Read the model definition and answer for the solid it produces. Units are mm, in the model's axes. Face numbers are marked on the shaded views. A direction names the side the tool comes from. Give positions to 0.01 mm unless a question says otherwise; leave off trailing zeros. Order: outer loops, then holes, each group sorted by start corner. A loop starts at its lowest first (then second) coordinate and runs counter-clockwise, first axis right, second up. Notation, with made-up numbers: (-36, -13.75) - (-24, -13.75) arc R28 cw to (-24, 24.25) - close; hole circle Ø8 at (62.25, 36.5). An arc over 180 degrees is marked (long way). Return JSON: item names as keys, results as strings.
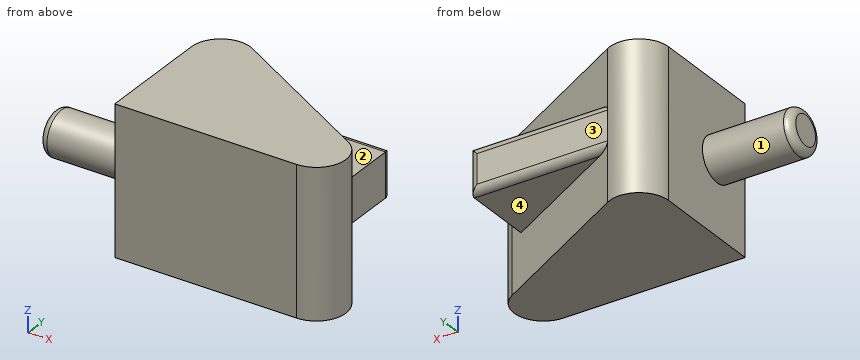
```python
from build123d import *

# Parameters (mm, degrees)
BOSS_EXTRUDE1_DEPTH = 5
SKETCH2_W           = 6.952682296
SKETCH2_H           = 2.551538718
SKETCH2_R           = 0.75
CUT_EXTRUDE1_DEPTH  = 3
SKETCH3_W           = 4.68163698
SKETCH3_H           = 1.5
BOSS_EXTRUDE2_DEPTH = 4.757403
FILLET1_R           = 0.25
FILLET2_R           = 0.25


with BuildPart() as part:
    # Sketch1 → Boss-Extrude1 (new body)
    with BuildSketch(Plane.XY):
        with BuildLine():
            Line((0, 2.17), (-3, 2.17))
            Line((-3, 2.17), (-3, 0.67))
            Line((-3, 0.67), (0, 0.67))
            Line((0, 0.67), (0, 0))
            Line((0, 0), (6.168897591, 0))
            ThreePointArc((6.168897591, 0), (7.13669318, 0.748262641), (6.656158202, 1.873256604))
            Line((6.656158202, 1.873256604), (1.487260611, 4.757403357))
            ThreePointArc((1.487260611, 4.757403357), (0.49367037, 4.74648677), (0, 3.884146753))
            Line((0, 3.884146753), (0, 2.17))
        make_face()
    extrude(amount=BOSS_EXTRUDE1_DEPTH)

    # Sketch2 → Cut-Extrude1 (cut)
    with BuildSketch(Plane.ZY.offset(3)):
        with Locations((2.401285903, 1.467822219)):
            Rectangle(SKETCH2_W, SKETCH2_H)
        with Locations((2.5, 1.42)):
            Circle(SKETCH2_R, mode=Mode.SUBTRACT)
    extrude(amount=-CUT_EXTRUDE1_DEPTH, mode=Mode.SUBTRACT)

    # Sketch3 → Boss-Extrude2 (add)
    with BuildSketch(Plane.XZ):
        with Locations((3.828079101, 2.5)):
            Rectangle(SKETCH3_W, SKETCH3_H)
    extrude(amount=-BOSS_EXTRUDE2_DEPTH)

    # Fillet1
    fillet1_edges = [part.edges().sort_by_distance(p)[0] for p in [
        (-3, 1.42, 1.75),
    ]]
    fillet(fillet1_edges, radius=FILLET1_R)

    # Fillet2
    fillet2_edges = [part.edges().sort_by_distance(p)[0] for p in [
        (3.828079101, 4.757403, 1.75),
        (3.828079101, 4.757403, 3.25),
        (6.168897591, 4.757403, 2.5),
    ]]
    fillet(fillet2_edges, radius=FILLET2_R)


solid = part.part
```
Q1. A cutting plane is placed at A-A (z = 1.3). Write down the section's boundary in (x, y).
Values:
{"outline": "(0, 0) - (6.17, 0) arc R1 ccw to (6.66, 1.87) - (1.49, 4.76) arc R1 ccw to (0, 3.88) - close"}
Q2. A cutting plane is placed at D-D (z = 2.5). Write down the section's boundary in (x, y).
Values:
{"outline": "(-3, 0.92) arc R0.25 ccw to (-2.75, 0.67) - (0, 0.67) - (0, 0) - (6.17, 0) arc R1 ccw to (6.66, 1.87) - (6.17, 2.15) - (6.17, 4.51) arc R0.25 ccw to (5.92, 4.76) - (1.49, 4.76) arc R1 ccw to (0, 3.88) - (0, 2.17) - (-2.75, 2.17) arc R0.25 ccw to (-3, 1.92) - close"}
Q3. Consider L1, parallel to Y at x = 4.5, z = 2.35; L2, parallel to X at y = 2.25, z = 1.9; L3, parallel to X at y = 2, z = 3.75. Determine where each line is inside the solid, lowest interval first.
Values:
{"L1": "y = 0 to 4.76", "L2": "x = 0 to 6.17", "L3": "x = 0 to 6.43"}
Q4. A cutting plane is placed at C-C (y = 1.42). Write down the section's boundary in (x, z).
Values:
{"outline": "(-3, 2) arc R0.25 ccw to (-2.75, 1.75) - (0, 1.75) - (0, 0) - (7.08, 0) - (7.08, 5) - (0, 5) - (0, 3.25) - (-2.75, 3.25) arc R0.25 ccw to (-3, 3) - close"}
Q5. A cutting plane is placed at B-B (x = 3.75). Write down the section's boundary in (y, z), and give its area (3 significant figures).
Values:
{"outline": "(0, 0) - (3.49, 0) - (3.49, 1.75) - (4.51, 1.75) arc R0.25 ccw to (4.76, 2) - (4.76, 3) arc R0.25 ccw to (4.51, 3.25) - (3.49, 3.25) - (3.49, 5) - (0, 5) - close", "area": "19.3 mm²"}
Q6. Given pin 1 (2 mm diameter, centred on x = 5, z = 2.5, fed in from +Y); pin 2 (1.2 mm diameter, centred on y = 4, z = 2.5, fed in from +X); pin 3 (1.2 mm diameter, centred on y = 2, z = 2, fed in from -X), each flat-ended and moving along its own axis, determine where each tip first touches the part or whether it passes through.
Values:
{"pin 1": "stops at y = 4.76", "pin 2": "stops at x = 6.17", "pin 3": "stops at x = -3"}
Q7. For the marked faces 1, 2, 3 and 4, determine the directions among +Z, -Z, +X, -X, +Y, -Y from which every point of the face is accessible in a straight line to the end or side of a thin tool.
Values:
{"face 1": "-X", "face 2": "+Z, +X, +Y", "face 3": "+Z, -Z, +X, +Y", "face 4": "-Z, +X, +Y"}
